from build123d import *

# Parameters (mm, degrees)
SKETCH2_W               = 11
SKETCH2_H               = 11
BOSS_EXTRUDE1_DEPTH     = 4
CUT_EXTRUDE2_DEPTH      = 9.746427842
CUT_EXTRUDE2_DEPTH_BACK = 9.746427842
SKETCH4_W               = 1
SKETCH4_H               = 1
SKETCH4_W_2             = 3
SKETCH4_H_2             = 1.012866832
CUT_EXTRUDE3_DEPTH      = 2.5
CUT_EXTRUDE3_DEPTH_BACK = 9.746427842
SKETCH5_R               = 2.25
SKETCH8_R               = 1
CUT_EXTRUDE4_DEPTH      = 1
SKETCH8_3_R             = 1
CUT_EXTRUDE5_DEPTH      = 0.55
FILLET2_R               = 0.5


with BuildPart() as part:
    # Sketch2 → Boss-Extrude1 (new body)
    with BuildSketch(Plane(origin=(0, 0, 0), x_dir=(1, 0, 0), z_dir=(0, 1, 0))):
        Rectangle(SKETCH2_W, SKETCH2_H)
    extrude(amount=BOSS_EXTRUDE1_DEPTH)

    # Sketch4 → Cut-Extrude2 (cut, two sides: drawn at the far end of the back side and taken through both)
    with BuildSketch(Plane(origin=(0, 0, 0), x_dir=(0, 0, -1), z_dir=(1, 0, 0)).offset(-CUT_EXTRUDE2_DEPTH_BACK)):
        with Locations((-3.5, 1.982791405)):
            Rectangle(SKETCH4_W, SKETCH4_H)
        with Locations((0, 1.989224821)):
            Rectangle(SKETCH4_W_2, SKETCH4_H_2)
        with Locations((3.5, 1.989224821)):
            Rectangle(SKETCH4_W, SKETCH4_H_2)
    extrude(amount=CUT_EXTRUDE2_DEPTH + CUT_EXTRUDE2_DEPTH_BACK, mode=Mode.SUBTRACT)

    # Sketch5 → Cut-Extrude3 (cut, two sides: drawn at the far end of the back side and taken through both)
    with BuildSketch(Plane(origin=(0, 0, 0), x_dir=(1, 0, 0), z_dir=(0, 1, 0)).offset(-CUT_EXTRUDE3_DEPTH_BACK)):
        with Locations(Location((0, 0, 0), (0, 0, 90))):
            Circle(SKETCH5_R)
    extrude(amount=CUT_EXTRUDE3_DEPTH + CUT_EXTRUDE3_DEPTH_BACK, mode=Mode.SUBTRACT)

    # Sketch8 → Cut-Extrude4 (cut)
    with BuildSketch(Plane(origin=(0, 0, 0), x_dir=(1, 0, 0), z_dir=(0, 1, 0))):
        with Locations(Location((0, -4, 0), (0, 0, 270))):
            Circle(SKETCH8_R)
    extrude(amount=CUT_EXTRUDE4_DEPTH, mode=Mode.SUBTRACT)

    # Sketch8_3 → Cut-Extrude5 (cut)
    with BuildSketch(Plane(origin=(0, 0, 0), x_dir=(1, 0, 0), z_dir=(0, 1, 0))):
        with Locations(Location((0, 4, 0), (0, 0, 270))):
            Circle(SKETCH8_3_R)
    extrude(amount=CUT_EXTRUDE5_DEPTH, mode=Mode.SUBTRACT)

    # Fillet2
    fillet2_edges = [part.edges().sort_by_distance(p)[0] for p in [
        (5.5, 4, 0),
        (0, 4, 5.5),
        (-5.5, 4, 0),
        (0, 4, -5.5),
    ]]
    fillet(fillet2_edges, radius=FILLET2_R)


solid = part.part
For this review, take the finished solid that the model builds, in its own axes (mm). A direction names the side the tool comes from. Coordinates: 2 decimals unless noted, no trailing zeros. Loops run counter-clockwise (first coordinate to the right, second up) from the corner with the lowest first, then second, coordinate; pieces in that order, holes last. Notation, with made-up numbers: (47, 15.25) -> (77, 15.25) arc R15 cw to (77, 29.25) -> close; hole circle Ø4 at (39, 59). An arc over 180 degrees is marked (long way). Write each question's results on one line, items separated by ' | '.
Q1. Machinability: for faces 4 (the flat face through (0, 4, 0)), 5 (the flat face through (0, 2, 4)), 6 (the cylindrical face through (0, 0.5, 3)), which of the approach directions +Z, -Z, +X, -X, +Y, -Y give a long, thin tool a straight path to every point of the face, cutting with its end or side? Answer none if there is none.
Taken from the geometry:
face 4: +Z, -Z, +X, -X, +Y | face 5: +X, -X | face 6: -Y
Q2. Add section B-B, the plane x = 0. State the section outline as (y, z) points, then the cut area to 3 significant figures.
Taken from the geometry:
outline: (0, -5.5) -> (3.5, -5.5) arc R0.5 ccw to (4, -5) -> (4, 5) arc R0.5 ccw to (3.5, 5.5) -> (0, 5.5) -> (0, 5) -> (1, 5) -> (1, 3) -> (0, 3) -> (0, 2.25) -> (2.5, 2.25) -> (2.5, -2.25) -> (0, -2.25) -> (0, -3) -> (0.55, -3) -> (0.55, -5) -> (0, -5) -> close; hole (1.48, -4) -> (2.5, -4) -> (2.5, -3) -> (1.48, -3) -> close; hole (1.48, 3) -> (2.48, 3) -> (2.48, 4) -> (1.48, 4) -> close | area: 27.5 mm²
Q3. To check wall thickness, follow line 1 along Z through (x, y) = (4.5, 1.55); line 2 along Y through (x, z) = (-4.25, -3.25); line 3 along X through (y, z) = (0.75, 4). State the ranges of each line that lie inside material, in increasing order. Write a range as [from, to].
Taken from the geometry:
line 1: [-5.5, -4], [-3, -1.5], [1.5, 3], [4, 5.5] | line 2: [0, 1.48], [2.5, 4] | line 3: [-5.5, -1], [1, 5.5]
Q4. Add section A-A, the plane y = 2.25. State the section outline as (x, z) points, then the cut area to 3 significant figures.
Taken from the geometry:
outline: (-5.5, -5.5) -> (5.5, -5.5) -> (5.5, -4) -> (-5.5, -4) -> close; (-5.5, -3) -> (5.5, -3) -> (5.5, -1.5) -> (1.68, -1.5) arc R2.25 cw to (-1.68, -1.5) -> (-5.5, -1.5) -> close; (-5.5, 1.5) -> (-1.68, 1.5) arc R2.25 cw to (1.68, 1.5) -> (5.5, 1.5) -> (5.5, 3) -> (-5.5, 3) -> close; (-5.5, 4) -> (5.5, 4) -> (5.5, 5.5) -> (-5.5, 5.5) -> close | area: 62.5 mm²
Q5. Mouldability with a two-part tool opening along Z and no side actions: class faces 1 (the flat face through (-5.5, 1, 0)), 2 (the flat face through (0, 2, 5.5)), 3 (the flat face through (-0.1, 2.496, -3.5)) as +Z half, -Z half, draft (parallel to the pull), parting line (faces both ways), or undercut.
Taken from the geometry:
face 1: draft | face 2: +Z half | face 3: undercut
Q6. Add section C-C, the plane z = 0. Count the separate pieces of the cut face and the enclosed holes in it, then the cut area to 3 significant figures.
Taken from the geometry:
separate pieces: 3 | enclosed holes: 0 | area: 26.1 mm²
Q7. Add section D-D, the plane x = -2.5. State the section outline as (y, z) points, then the cut area to 3 significant figures.
Taken from the geometry:
outline: (0, -5.5) -> (3.5, -5.5) arc R0.5 ccw to (4, -5) -> (4, 5) arc R0.5 ccw to (3.5, 5.5) -> (0, 5.5) -> close; hole (1.48, -4) -> (2.5, -4) -> (2.5, -3) -> (1.48, -3) -> close; hole (1.48, -1.5) -> (2.5, -1.5) -> (2.5, 1.5) -> (1.48, 1.5) -> close; hole (1.48, 3) -> (2.48, 3) -> (2.48, 4) -> (1.48, 4) -> close | area: 38.8 mm²
Q8. For pin 1 Ø0.8 at (x, z) = (0, -3.5) entering from -Y, flat-tipped, find the tip position at first contact; note if it passes through.
Taken from the geometry:
pin 1: y = 0.55
